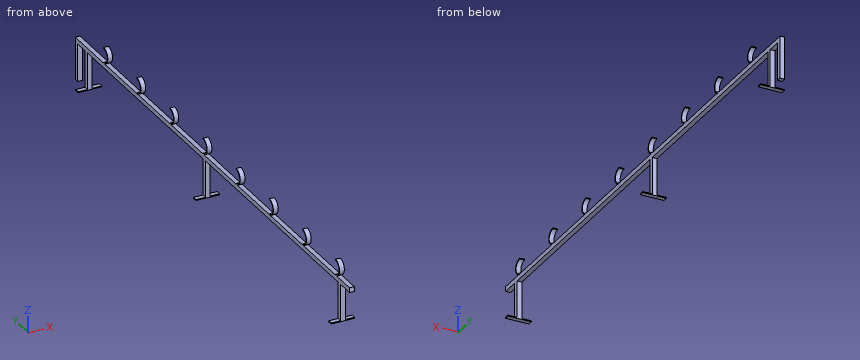
Autodesk Inventor part; units mm, degrees
ref_plane "YZ Plane" through (0, 0, 0) normal (1, 0, 0) x (0, 1, 0)
ref_plane "XZ Plane" through (0, 0, 0) normal (0, 1, 0) x (-1, 0, 0)
ref_plane "XY Plane" through (0, 0, 0) normal (0, 0, 1) x (1, 0, 0)
sketch "Sketch1" plane through (0, 0, 0) normal (0, 0, 1) x (1, 0, 0)
  line L0 (0, 0) -> (25, 0)
  line L1 (25, 0) -> (25, 2800)
  line L2 (25, 2800) -> (0, 2800)
  line L3 (0, 2800) -> (0, 0)
  dimension "d0" = 25
  dimension "d1" = 2800
extrude "Extrusion1" add sketch "Sketch1" along normal blind 25
sketch "Sketch2" plane through (0, 0, 0) normal (0, 0, -1) x (-1, 0, 0)
  line L0 (-25, 0) -> (-25, 2800)
  line L1 (0, 2800) -> (0, 0)
  line L2 (-25, 2800) -> (0, 2800)
  line L3 (0, 2800) -> (0, 2775)
  line L4 (0, 2775) -> (-25, 2775)
  line L5 (-25, 2775) -> (-25, 2800)
  dimension "d4" = 25
extrude "Extrusion2" add sketch "Sketch2" along normal blind 200
sketch "Sketch6" plane through (0, 0, 25) normal (-1, 0, 0) x (0, 0, 1)
  line L0 (-225, 2775) -> (-225, 2800)
  line L1 (-225, 2675) -> (-220, 2675)
  line L2 (-220, 2675) -> (-220, 2700)
  line L3 (-220, 2700) -> (-225, 2700)
  line L4 (-225, 2700) -> (-225, 2675)
  point P0 (-25, 0)
  dimension "d13" = 5
  dimension "d14" = 25
extrude "Extrusion5" add sketch "Sketch6" along normal blind 50 and the other way blind 75
sketch "Sketch7" plane through (0, 0, 25) normal (-1, 0, 0) x (0, 0, 1)
  line L0 (-225, 1496) -> (-225, 1471)
  line L1 (-25, 1471) -> (-225, 1471)
  line L2 (-225, 1496) -> (-220, 1496)
  line L3 (-220, 1496) -> (-220, 1471)
  line L4 (-220, 1471) -> (-225, 1471)
  line L5 (-225, 1471) -> (-225, 1496)
  point P0 (-25, 0)
  dimension "d22" = 5
extrude "Extrusion6" add sketch "Sketch7" along normal blind 50 and the other way blind 75
sketch "Sketch8" plane through (0, 0, 25) normal (-1, 0, 0) x (0, 0, 1)
  arc A0 (-0.0707, 2510) -> (83.9293, 2510) centre (41.9293, 2510) ccw
  arc A1 (3.9293, 2510) -> (79.9293, 2510) centre (41.9293, 2510) ccw
  line L0 (-0.0707, 2510) -> (3.9293, 2510)
  line L1 (0, 0) -> (0, 2800)
  line L2 (79.9293, 2510) -> (83.9293, 2510)
  line L3 (0, 2800) -> (0, 0)
  line L4 (0, 2800) -> (42, 2800)
  point P0 (-25, 0)
  dimension "d31" = 4
  dimension "d39" = 42
  dimension "d40" = 290
extrude "Extrusion7" add sketch "Sketch8" against normal up to surface (25 mm away)
pattern_linear "Rectangular Pattern3" count 8 spacing 338 along (0, -1, 0) of "Extrusion7"
sketch "Sketch10" plane through (0, 2800, -200) normal (-1, 0, 0) x (0, 0, 1)
  line L0 (200, -2800) -> (225, -2800)
  line L1 (225, -2800) -> (267, -2800)
  dimension "d41" = 42
sketch "Sketch11" plane through (-50, 2700, -195) normal (0, 0, 1) x (1, 0, 0)
  line L0 (75, 0) -> (50, 0)
  line L1 (50, 0) -> (50, -25)
  line L2 (50, -25) -> (75, -25)
  line L3 (75, -25) -> (75, 0)
  line L4 (75, 0) -> (50, -25) construction
  line L5 (50, 0) -> (75, -25) construction
  line L6 (125, -25) -> (0, -25)
  point P0 (50, -2700)
  point P1 (62.5, -12.5)
  dimension "d42" = 25
  dimension "d43" = 25
  dimension "d49" = 0
extrude "Extrusion8" add sketch "Sketch11" along normal up to next
pattern_linear "Rectangular Pattern4" count 2 spacing 1204 along (0, -1, 0) of "Extrusion8"
pattern_linear "Rectangular Pattern5" count 2 spacing 1379 along (0, -1, 0) of "Extrusion6"
sketch "Sketch12" plane through (-50, 117, -195) normal (0, 0, 1) x (1, 0, 0)
  line L0 (50, 0) -> (75, 0)
  line L1 (75, 0) -> (75, -25)
  line L2 (75, -25) -> (50, -25)
  line L3 (50, -25) -> (50, 0)
  line L4 (50, 0) -> (75, -25) construction
  line L5 (75, 0) -> (50, -25) construction
  line L6 (125, -25) -> (0, -25)
  point P0 (50, -117)
  point P1 (62.5, -12.5)
  dimension "d53" = 25
  dimension "d54" = 25
  dimension "d55" = 0
extrude "Extrusion9" add sketch "Sketch12" along normal up to next
properties part number "Stand"
Read the model definition and answer for the solid it produces. Units are mm, in the model's axes. Round coordinates to 2 decimals unless told otherwise and drop trailing zeros. Write each loop counter-clockwise with the first axis right and the second up, starting at its lowest first coordinate (ties: lowest second). Pieces come first, ordered by that corner, then holes. Notation, with made-up numbers: (89, 19.25) - (148, 19.25) arc R20 ccw to (148, 56.25) - close; hole circle Ø1 at (0, 57.5). An arc over 180 degrees is marked (long way). Use a Markdown table: item, result.
(1) The part is cut by section B-B (y = 1404.5). Write down the section's boundary in (x, z).
Reported:
| item | result |
|---|---|
| outline | (0, 0) - (25, 0) - (25, 25) - (0, 25) - close |
(2) Straight lines are drawn through the part: line 1 along Y through (x, z) = (23, -69.5); line 2 along Z through (x, y) = (2, 2631.5). For each, find the intervals that lie inside material, in ascending order. Write a range as [from, to].
Reported:
| item | result |
|---|---|
| line 1 | [92, 117], [1471, 1496], [2675, 2700], [2775, 2800] |
| line 2 | [0, 25] |
(3) Each of these flat-tipped pins is pushed along its axis until it touches: pin 1 Ø12 at (x, y) = (21, 2120) entering from +Z; pin 2 Ø2 at (x, z) = (15, 107.5) entering from +Y; pin 3 Ø10 at (x, z) = (11, -141.5) entering from -Y. Where does it stop, or does it pass through?
Reported:
| item | result |
|---|---|
| pin 1 | z = 25 |
| pin 2 | y = 2510 |
| pin 3 | y = 92 |
(4) The part is cut by section A-A (z = -33.5). Write down the section's boundary in (x, y), then the cut area to 3 significant figures.
Reported:
| item | result |
|---|---|
| outline | (0, 92) - (25, 92) - (25, 117) - (0, 117) - close; (0, 1471) - (25, 1471) - (25, 1496) - (0, 1496) - close; (0, 2675) - (25, 2675) - (25, 2700) - (0, 2700) - close; (0, 2775) - (25, 2775) - (25, 2800) - (0, 2800) - close |
| area | 2,500 mm2 |
